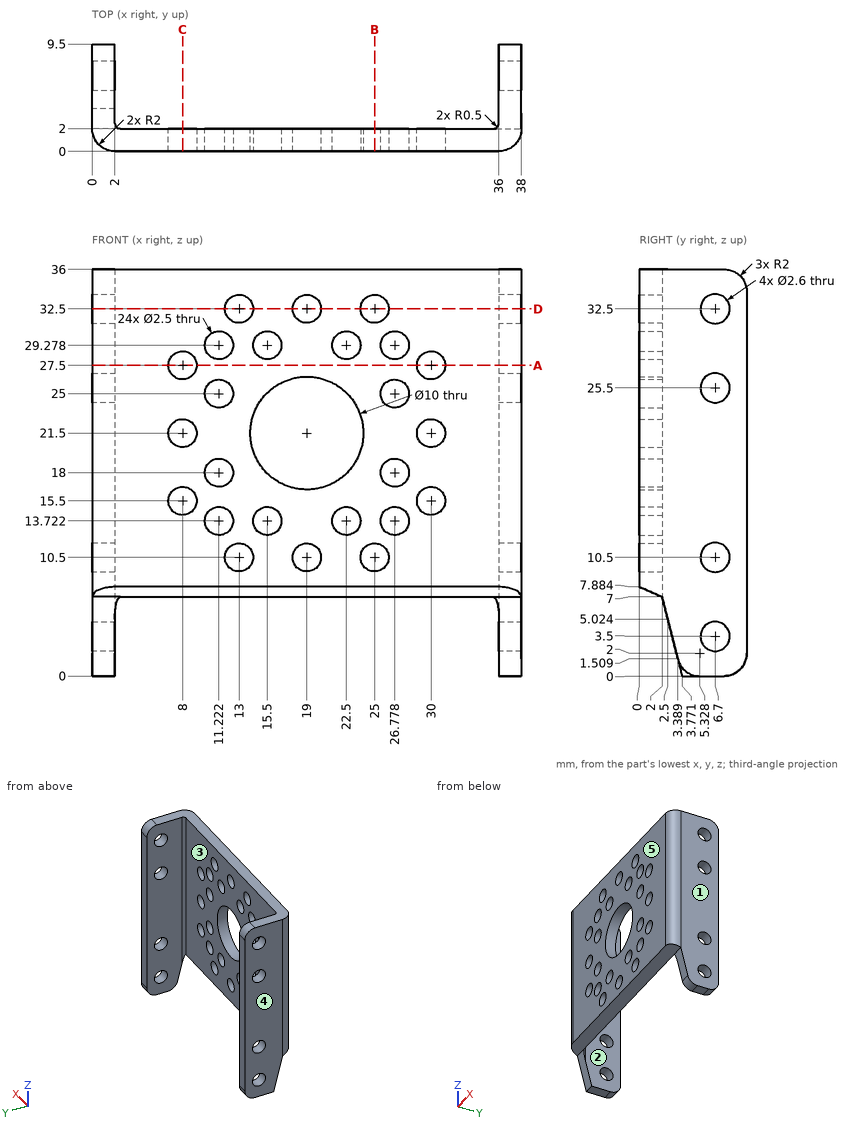
Job drawing, mm, ordinate dimensions from the low corner. One solid piece. A direction names the side the tool comes from. Round coordinates to 2 decimals unless told otherwise and drop trailing zeros. Write each loop counter-clockwise with the first axis right and the second up, starting at its lowest first coordinate (ties: lowest second). Pieces come first, ordered by that corner, then holes. Notation, with made-up numbers: (52.25, -20.5) -> (96.25, -20.5) arc R26 ccw to (96.25, 16.5) -> close; hole circle Ø10 at (25.25, 21.25). An arc over 180 degrees is marked (long way). Answer as CSV lines item,"result".
1. Tool access for the marked faces 1 and 2: list every direction of +Z, -Z, +X, -X, +Y, -Y with a clear straight run to the whole face (end or side of a thin tool).
Resolved:
face 1,"+Z, -Z, +X, +Y, -Y"
face 2,"+Z, -Z, +Y"
2. Slice it at C-C, the plane x = 8. List the corners of the cut face in (y, z).
Resolved:
outline,"(0, 7.88) -> (2, 7) -> (2, 14.25) -> (0, 14.25) -> close; (0, 16.75) -> (2, 16.75) -> (2, 20.25) -> (0, 20.25) -> close; (0, 22.75) -> (2, 22.75) -> (2, 26.25) -> (0, 26.25) -> close; (0, 28.75) -> (2, 28.75) -> (2, 36) -> (0, 36) -> close"
3. Pin check, flat tips, straight feed: pin 1 Ø3 at (x, z) = (11.22, 18) entering from -Y; pin 2 Ø13 at (x, z) = (19, 21.5) entering from +Y. Stop position of each tip, or through.
Resolved:
pin 1,"y = 0"
pin 2,"y = 2"
4. Slice it at A-A, the plane z = 27.5. List the corners of the cut face in (x, y).
Resolved:
outline,"(0, 2) arc R2 ccw to (2, 0) -> (6.75, 0) -> (6.75, 2) -> (2.5, 2) arc R0.5 cw to (2, 2.5) -> (2, 9.5) -> (0, 9.5) -> close; (9.25, 0) -> (28.75, 0) -> (28.75, 2) -> (9.25, 2) -> close; (31.25, 0) -> (36, 0) arc R2 ccw to (38, 2) -> (38, 9.5) -> (36, 9.5) -> (36, 2.5) arc R0.5 cw to (35.5, 2) -> (31.25, 2) -> close"
5. Drill centre lines: line 1 (Z direction, x = 8, y = 0.6); line 2 (Z direction, x = 22.5, y = 0.8); line 3 (X direction, y = 7.25, z = 16). Where is each one in solid material? Low to high.
Resolved:
line 1,"7.62 to 14.25, 16.75 to 20.25, 22.75 to 26.25, 28.75 to 36"
line 2,"7.53 to 12.47, 14.97 to 17.93, 25.07 to 28.03, 30.53 to 36"
line 3,"0 to 2, 36 to 38"
6. Mould opens along X. For the marked faces 3, 4 and 5 say: +X half, -X half, draft (parallel to the pull), parting line (faces both ways), or undercut.
Resolved:
face 3,"undercut"
face 4,"-X half"
face 5,"draft"
7. Slice it at D-D, the plane z = 32.5. State how many separate pieces and enclosed holes the cut face has.
Resolved:
separate pieces,"6"
enclosed holes,"0"
8. Slice it at B-B, the plane x = 25. List the corners of the cut face in (y, z).
Resolved:
outline,"(0, 7.88) -> (2, 7) -> (2, 9.25) -> (0, 9.25) -> close; (0, 11.75) -> (2, 11.75) -> (2, 31.25) -> (0, 31.25) -> close; (0, 33.75) -> (2, 33.75) -> (2, 36) -> (0, 36) -> close"
